from build123d import *

# Parameters (mm, degrees)
SKETCH2_R          = 2.5
CUT_EXTRUDE1_DEPTH = 20


with BuildPart() as part:
    # Sketch1 → Revolve1 (revolve)
    with BuildSketch(Plane.XY, mode=Mode.PRIVATE) as revolve1_sk:
        Polygon((0, 325.102863253), (0, 271.755588021), (15, 271.755588021), align=None)
    revolve(revolve1_sk.sketch.rotate(Axis((0, 0, 0), (0, 1, 0)), 90), axis=Axis((0, 0, 0), (0, 1, 0)))

    # Sketch2 → Cut-Extrude1 (cut)
    with BuildSketch(Plane.XZ.offset(-271.755588021)):
        with Locations(Location((0, 0, 0), (0, 0, 270))):
            Circle(SKETCH2_R)
    extrude(amount=-CUT_EXTRUDE1_DEPTH, mode=Mode.SUBTRACT)

    # Sketch4 → Cut-Revolve1 (revolve, cut)
    with BuildSketch(Plane.XY, mode=Mode.PRIVATE) as cut_revolve1_sk:
        Polygon((15, 271.755588021), (0, 325.102863253), (0, 321.408464024), (13.961221764, 271.755588021), align=None)
    revolve(cut_revolve1_sk.sketch.rotate(Axis((0, 271.755588021, 0), (0, 1, 0)), 90), axis=Axis((0, 271.755588021, 0), (0, 1, 0)), mode=Mode.SUBTRACT)


solid = part.part
Read the model definition and answer for the solid it produces. Units are mm, in the model's axes. Round coordinates to 2 decimals unless told otherwise and drop trailing zeros. Write each loop counter-clockwise with the first axis right and the second up, starting at its lowest first coordinate (ties: lowest second). Pieces come first, ordered by that corner, then holes.
Q1. Find section A-A on y = 316.5. Determine the outline of the cut face in (x, z).
Values:
outline: circle Ø2.76 at (0, 0)
Q2. Flat-ended cylindrical pins translate along their axes: P1, Ø6, axis at y = 283.5, z = 2, coming from the +X side; P2, Ø12, axis at x = 2, z = -5.5, coming from the +Y side; P3, Ø1.5, axis at y = 315, z = 3, coming from the -X side; P4, Ø1.5, axis at y = 303, z = -5.5, coming from the +X side. Find the tip coordinate at first contact, or state that the pin passes through.
Values:
P1: stops at x = 11.41
P2: stops at y = 321.41
P3: passes through
P4: stops at x = 2.14
Q3. Straight lines are drawn through the part: line 1 (X direction, y = 286, z = 0); line 2 (X direction, y = 278.5, z = 0); line 3 (X direction, y = 308.5, z = -0.75). For each, find the intervals that lie inside material, in ascending order.
Values:
line 1: x = -9.96 to -2.5, 2.5 to 9.96
line 2: x = -12.06 to -2.5, 2.5 to 12.06
line 3: x = -3.55 to 3.55
Q4. The mould has two halves that part along X. Classify faces 1 (the face through (-2.44, 281.62, 0.54)), 2 (the face through (0, 291.756, 0)), 3 (the face through (-2.13, 296.23, -6.75)), 4 (the face through (0, 271.756, 3)): released by +X, released by -X, zero draft, split by the parting line, or undercut.
Values:
face 1: undercut
face 2: undercut
face 3: split by the parting line
face 4: zero draft
